The model under review builds one solid part; all positions refer to its coordinate system, in mm. Give positions to 0.01 mm unless a question says otherwise; leave off trailing zeros. Loops run counter-clockwise (first coordinate to the right, second up) from the corner with the lowest first, then second, coordinate; pieces in that order, holes last. Notation, with made-up numbers: M -2,-25.5 L 18,-25.5 A22 cw 18,-12.5 Z; hole C 0,-37.5 d9. An arc over 180 degrees is marked long. Return JSON: item names as keys, results as strings.
```python
from build123d import *

# Parameters (mm, degrees)
SKETCH_1_W          = 23
SKETCH_1_H          = 6
EXTRUDE_1_DEPTH     = 5
SKETCH_2_R          = 1.6
CUT_EXTRUDE_1_DEPTH = 5
FILLET_1_R          = 1


with BuildPart() as part:
    # 草图1 → 凸台-拉伸1 (new body)
    with BuildSketch(Plane.XY):
        Rectangle(SKETCH_1_W, SKETCH_1_H)
    extrude(amount=EXTRUDE_1_DEPTH)

    # 草图2 → 切除-拉伸1 (cut)
    with BuildSketch(Plane.XY.offset(5)):
        with Locations((-7, 0)):
            Circle(SKETCH_2_R)
        with Locations((7, 0)):
            Circle(SKETCH_2_R)
        with Locations((0, -0.4)):
            Circle(SKETCH_2_R)
    extrude(amount=-CUT_EXTRUDE_1_DEPTH, mode=Mode.SUBTRACT)

    # 圆角1
    fillet_1_edges = [part.edges().sort_by_distance(p)[0] for p in [
        (11.5, -3, 2.5),
        (-11.5, -3, 2.5),
        (-11.5, 3, 2.5),
        (11.5, 3, 2.5),
    ]]
    fillet(fillet_1_edges, radius=FILLET_1_R)


solid = part.part
```
1) Consider section C-C on y = 0.75. Write out the cut boundary in (x, z).
From the geometry:
{"outline": "M -11.5,0 L -8.41,0 L -8.41,5 L -11.5,5 Z; M -5.59,0 L -1.11,0 L -1.11,5 L -5.59,5 Z; M 1.11,0 L 5.59,0 L 5.59,5 L 1.11,5 Z; M 8.41,0 L 11.5,0 L 11.5,5 L 8.41,5 Z"}
2) Consider section D-D on x = -6. Write out the cut boundary in (y, z).
From the geometry:
{"outline": "M -3,0 L -1.25,0 L -1.25,5 L -3,5 Z; M 1.25,0 L 3,0 L 3,5 L 1.25,5 Z"}
3) The part is to be moulded in two halves that separate along X. For faces 1 (the face through (0, -2, 3)), 2 (the face through (11.199, 2.715, 2.535)), 3 (the face through (0, -3, 2)), say which applies: released by +X, released by -X, zero draft, split by the parting line, or undercut.
From the geometry:
{"face 1": "undercut", "face 2": "released by +X", "face 3": "zero draft"}
4) Consider section B-B on z = 4.4. Write out the cut boundary in (x, y), then the cut area to 3 significant figures.
From the geometry:
{"outline": "M -11.5,-2 A1 ccw -10.5,-3 L 10.5,-3 A1 ccw 11.5,-2 L 11.5,2 A1 ccw 10.5,3 L -10.5,3 A1 ccw -11.5,2 Z; hole C -7,0 d3.2; hole C 0,-0.4 d3.2; hole C 7,0 d3.2", "area": "113 mm²"}
5) Wall thickness on L1, parallel to X at y = -1, z = 0.9; L2, parallel to Y at x = -7, z = 3.5; L3, parallel to Y at x = 0, z = 4.45: over which ranges is each line inside the solid? List them lowest first. Write a range as from..to.
From the geometry:
{"L1": "-11.5..-8.25, -5.75..-1.48, 1.48..5.75, 8.25..11.5", "L2": "-3..-1.6, 1.6..3", "L3": "-3..-2, 1.2..3"}
6) Consider section A-A on x = 7. Write out the cut boundary in (y, z).
From the geometry:
{"outline": "M -3,0 L -1.6,0 L -1.6,5 L -3,5 Z; M 1.6,0 L 3,0 L 3,5 L 1.6,5 Z"}
